Check sheet for the drawn part. Datum: minimum x, y, z corner. Units: mm. A direction names the side the tool comes from. Round coordinates to 2 decimals unless told otherwise and drop trailing zeros. Loops run counter-clockwise (first coordinate to the right, second up) from the corner with the lowest first, then second, coordinate; pieces in that order, holes last. Notation, with made-up numbers: (47.5, 12.25) -> (98.5, 12.25) arc R24 ccw to (98.5, 29.25) -> close; hole circle Ø5 at (-31, 6.25). An arc over 180 degrees is marked (long way). Write item = value, one per line. Start each with the question number.
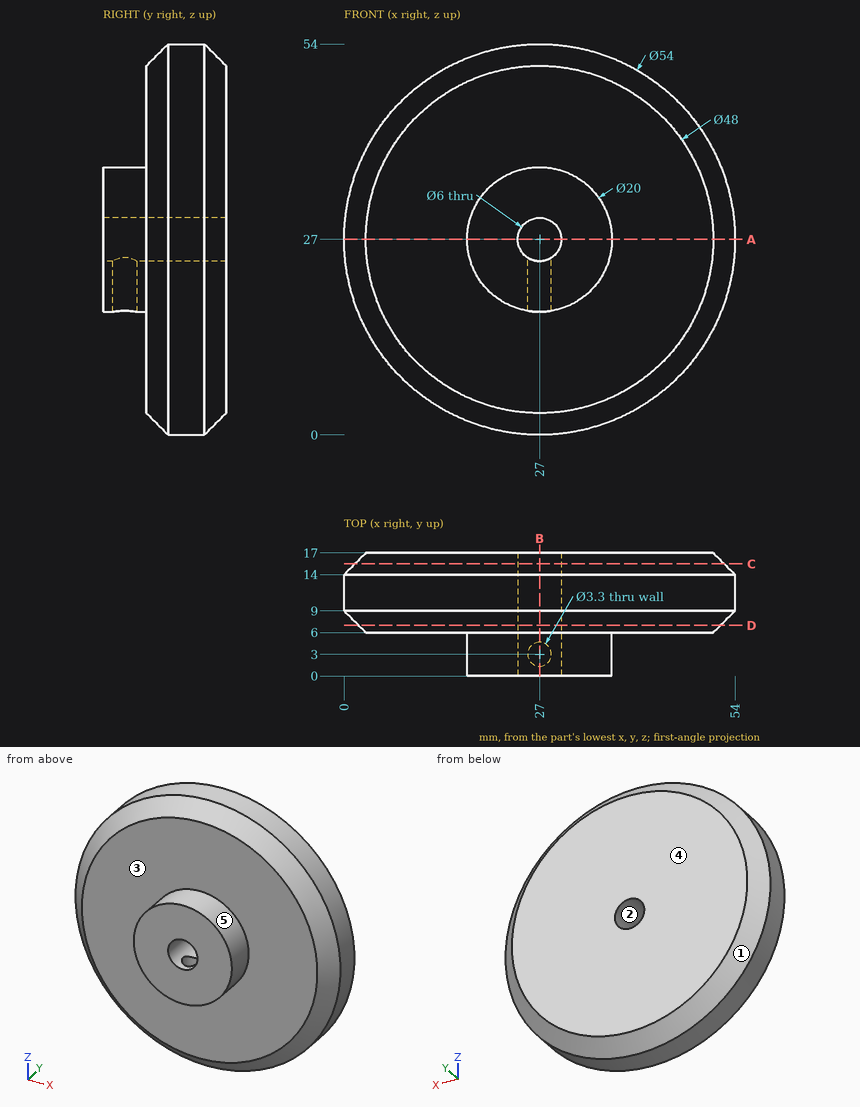
(1) Section check C-C on y = 15.5. Enter the section's corners in (x, z).
(2) Depth check by flat-ended pin: pin 1 Ø2 at (y, z) = (8, 38) entering from -X; pin 2 Ø5 at (x, z) = (27, 27) entering from +Y; pin 3 Ø5 at (y, z) = (2, 30) entering from -X; pin 4 Ø4.5 at (x, y) = (27, 3) entering from +Z. Enter the tip coordinate at first touch or a pass-through.
(3) Access from +Z, -Z, +X, -X, +Y, -Y to the whole of each face (thin tool, end or side, straight path). Record for the marked faces 4 and 5.
(4) Section check D-D on y = 7. Enter the section's corners in (x, z), then the cut area to 3 significant figures.
(5) Scan lines: line 1 (Y direction, x = 27, z = 23.25); line 2 (Y direction, x = 19.5, z = 42); line 3 (Z direction, x = 10, y = 13). Record each from-to range of solid material in increasing order. Write a range as [from, to].
(6) Section check A-A on z = 27. Enter the section's corners in (x, y).
(7) Section check B-B on x = 27. Enter the section's corners in (y, z).
(8) Draft check along Z on the marked faces 1, 2 and 3. Enter one of: +Z half, -Z half, draft (parallel to the pull), parting line (faces both ways), or undercut.
Computed values:
q1.outline = circle Ø51 at (27, 27); hole circle Ø6 at (27, 27)
q2.pin_1 = 2.26
q2.pin_2 = through
q2.pin_3 = 17.01
q2.pin_4 = 37
q3.face_4 = +Z, -Z, +X, -X, +Y
q3.face_5 = -Y
q4.outline = circle Ø50 at (27, 27); hole circle Ø6 at (27, 27)
q4.area = 1,940 mm²
q5.line_1 = [0, 1.35], [4.65, 17]
q5.line_2 = [6, 17]
q5.line_3 = [6.02, 47.98]
q6.outline = (0, 9) -> (3, 6) -> (17, 6) -> (17, 0) -> (24, 0) -> (24, 17) -> (3, 17) -> (0, 14) -> close; (30, 0) -> (37, 0) -> (37, 6) -> (51, 6) -> (54, 9) -> (54, 14) -> (51, 17) -> (30, 17) -> close
q7.outline = (0, 17) -> (1.35, 17) -> (1.35, 24) -> (0, 24) -> close; (0, 30) -> (17, 30) -> (17, 51) -> (14, 54) -> (9, 54) -> (6, 51) -> (6, 37) -> (0, 37) -> close; (4.65, 17) -> (6, 17) -> (6, 3) -> (9, 0) -> (14, 0) -> (17, 3) -> (17, 24) -> (4.65, 24) -> close
q8.face_1 = parting line
q8.face_2 = undercut
q8.face_3 = draft
